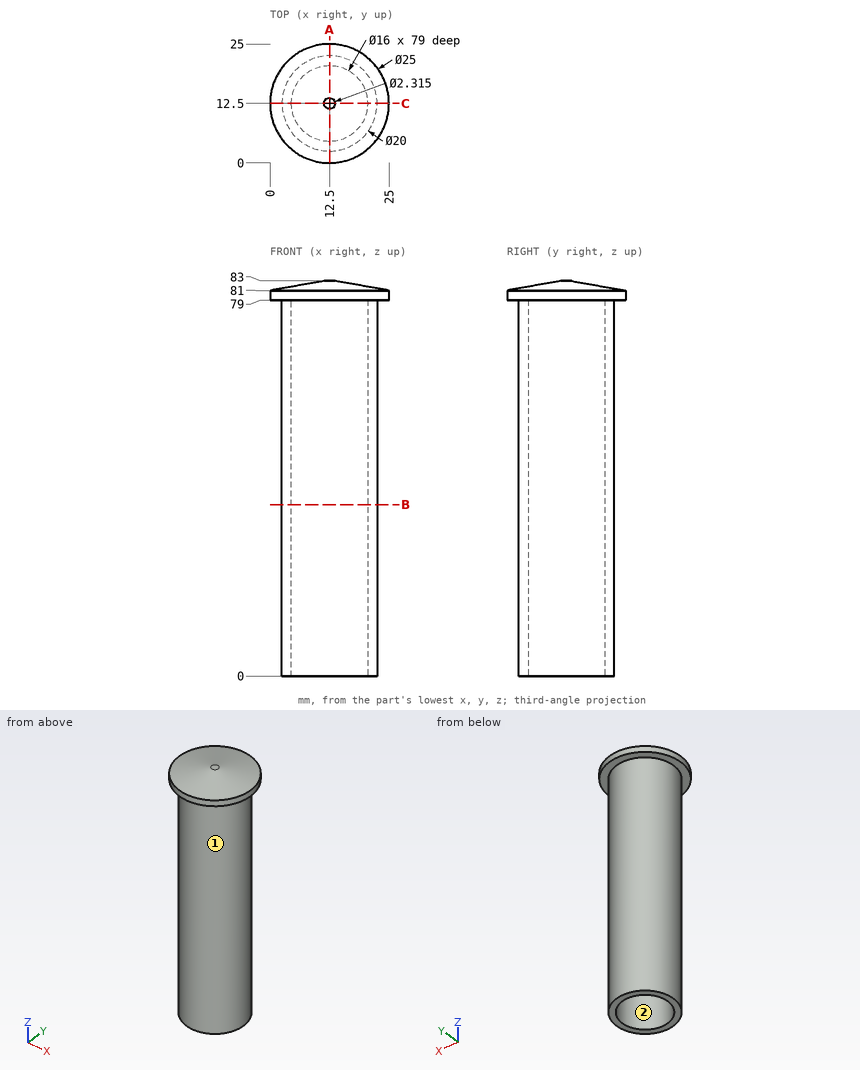
The drawing under review shows one solid part. Ordinate dimensions are in mm from its lowest x, y, z. Round coordinates to 2 decimals unless told otherwise and drop trailing zeros. Loops run counter-clockwise (first coordinate to the right, second up) from the corner with the lowest first, then second, coordinate; pieces in that order, holes last. Notation, with made-up numbers: (6, 3) - (33, 3) arc R22 cw to (33, 34) - close; hole circle Ø4 at (-35.5, 5). An arc over 180 degrees is marked (long way). Put each result on its own line as item: value. Start each with the question number.
1. Consider section A-A on x = 12.5. State the section outline as (y, z) points.
2. Consider section B-B on z = 36. State the section outline as (x, y) points.
3. Mouldability with a two-part tool opening along X and no side actions: class the marked faces 1 and 2 as +X half, -X half, draft (parallel to the pull), parting line (faces both ways), or undercut.
4. Insertion check: P1, Ø12, axis at y = 4, z = 16.5, coming from the -X side; P2, Ø6, axis at x = 17, z = 38.5, coming from the -Y side; P3, Ø14.5, axis at x = 12.5, y = 12.5, coming from the -Z side. Each pin has a flat end and moves straight along its axis. Give the tip position at first contact, or say it passes through.
5. For probe 1 along X at (y, z) = (12.75, 6.5); probe 2 along Y at (x, z) = (10.25, 41), list the stretches that pass through material, from the lowest coordinate up. Write a range as [from, to].
Result sheet:
1. outline: (0, 79) - (2.5, 79) - (2.5, 0) - (4.5, 0) - (4.5, 79) - (20.5, 79) - (20.5, 0) - (22.5, 0) - (22.5, 79) - (25, 79) - (25, 81) - (13.66, 83) - (11.34, 83) - (0, 81) - close
2. outline: circle Ø20 at (12.5, 12.5); hole circle Ø16 at (12.5, 12.5)
3. face 1: parting line
3. face 2: undercut
4. P1: x = 2.82
4. P2: y = 2.61
4. P3: z = 79
5. probe 1: [2.5, 4.5], [20.5, 22.5]
5. probe 2: [2.76, 4.82], [20.18, 22.24]
